Verification items for the finished model (mm, model axes). Coordinates: 2 decimals unless noted, no trailing zeros. Loops run counter-clockwise (first coordinate to the right, second up) from the corner with the lowest first, then second, coordinate; pieces in that order, holes last.
Q1. Sectioned sample at B-B (z = 13.5). Enter the section's corners in (x, y), then the cut area to 3 significant figures.
Q2. Sectioned sample at A-A (x = -22.5). Enter the section's corners in (y, z), then the cut area to 3 significant figures.
Q3. Material ranges on probe 1 along Z at (x, y) = (-3, 1.65); probe 2 along X at (y, z) = (1, -12.5); probe 3 along X at (y, z) = (1.75, 16), recorded low to high.
Q4. Go/stop test with flat-tipped pins: P1, Ø0.5, axis at y = 1.5, z = 18, coming from the +X side; P2, Ø0.6, axis at x = -33, y = 0.5, coming from the -Z side; P3, Ø1, axis at y = 0.5, z = 7.5, coming from the -X side. Record where each tip stops, or that it passes through.
Autodesk Inventor part; units mm, degrees
ref_plane "YZ Plane" through (0, 0, 0) normal (1, 0, 0) x (0, 1, 0)
ref_plane "XZ Plane" through (0, 0, 0) normal (0, 1, 0) x (-1, 0, 0)
ref_plane "XY Plane" through (0, 0, 0) normal (0, 0, 1) x (1, 0, 0)
sketch "Эскиз1" plane through (0, 0, 0) normal (0, 1, 0) x (-1, 0, 0)
  line L0 (-34.5, 19) -> (34.5, 19)
  line L1 (34.5, 19) -> (34.5, -19)
  line L2 (34.5, -19) -> (-34.5, -19)
  line L3 (-34.5, -19) -> (-34.5, 19)
  line L4 (-34.5, 19) -> (34.5, -19) construction
  line L5 (34.5, 19) -> (-34.5, -19) construction
  line L6 (34.5, -9.5) -> (34.5, 9.5)
  line L7 (36.5, -15.5) -> (32.5, -15.5)
  line L8 (32.5, -15.5) -> (32.5, -3.5)
  line L9 (32.5, -3.5) -> (36.5, -3.5)
  line L10 (36.5, -3.5) -> (36.5, -15.5)
  line L11 (36.5, -15.5) -> (32.5, -3.5) construction
  line L12 (32.5, -15.5) -> (36.5, -3.5) construction
  line L13 (36.5, 3.5) -> (32.5, 3.5)
  line L14 (32.5, 3.5) -> (32.5, 15.5)
  line L15 (32.5, 15.5) -> (36.5, 15.5)
  line L16 (36.5, 15.5) -> (36.5, 3.5)
  line L17 (36.5, 3.5) -> (32.5, 15.5) construction
  line L18 (32.5, 3.5) -> (36.5, 15.5) construction
  line L19 (-34.5, -9.5) -> (-34.5, 9.5)
  line L20 (-32.5, -15.5) -> (-36.5, -15.5)
  line L21 (-36.5, -15.5) -> (-36.5, -3.5)
  line L22 (-36.5, -3.5) -> (-32.5, -3.5)
  line L23 (-32.5, -3.5) -> (-32.5, -15.5)
  line L24 (-32.5, -15.5) -> (-36.5, -3.5) construction
  line L25 (-36.5, -15.5) -> (-32.5, -3.5) construction
  line L26 (-32.5, 3.5) -> (-36.5, 3.5)
  line L27 (-36.5, 3.5) -> (-36.5, 15.5)
  line L28 (-36.5, 15.5) -> (-32.5, 15.5)
  line L29 (-32.5, 15.5) -> (-32.5, 3.5)
  line L30 (-32.5, 3.5) -> (-36.5, 15.5) construction
  line L31 (-36.5, 3.5) -> (-32.5, 15.5) construction
  point P0 (0, 0)
  point P1 (34.5, 0)
  point P2 (-34.5, 0)
  point P3 (-34.5, 15.5)
  point P4 (-34.5, 3.5)
  point P5 (-34.5, -3.5)
  point P6 (-34.5, -15.5)
  point P7 (34.5, -15.5)
  point P8 (34.5, -3.5)
  point P9 (34.5, 3.5)
  point P10 (34.5, 15.5)
  dimension "d0" = 69
  dimension "d1" = 38
  dimension "d4" = 19
  dimension "d5" = 4
  dimension "d6" = 12
  dimension "d7" = 4
  dimension "d8" = 12
  dimension "d9" = 19
  dimension "d10" = 4
  dimension "d11" = 12
  dimension "d12" = 4
  dimension "d13" = 12
extrude "Выдавливание1" add sketch "Эскиз1" along normal blind 2 contours L0 L1 L15 L14 L13 L9 L8 L7 L2 L3 L20 L23 L22 L26 L29 L28
fillet "Сопряжение1" radius 0.5 8 edges at (-32.5, 1, -3.5) (-32.5, 1, -15.5) (-32.5, 1, 3.5) (-32.5, 1, 15.5) (32.5, 1, -15.5) (32.5, 1, -3.5) (32.5, 1, 3.5) (32.5, 1, 15.5)
fillet "Сопряжение2" radius 1 8 edges at (34.5, 1, -3.5) (34.5, 1, 3.5) (34.5, 1, -15.5) (34.5, 1, 15.5) (-34.5, 1, -15.5) (-34.5, 1, -3.5) (-34.5, 1, 3.5) (-34.5, 1, 15.5)
fillet "Сопряжение3" radius 2 4 edges at (-34.5, 1, -19) (-34.5, 1, 19) (34.5, 1, -19) (34.5, 1, 19)
sketch "Эскиз2" plane through (0, 2, 0) normal (0, 1, 0) x (1, 0, 0)
  line L0 (-34.5, -19) -> (34.5, -19)
  line L1 (34.5, -19) -> (34.5, 19)
  line L2 (34.5, 19) -> (-34.5, 19)
  line L3 (-34.5, 19) -> (-34.5, -19)
  line L4 (-34.5, -19) -> (34.5, 19) construction
  line L5 (34.5, -19) -> (-34.5, 19) construction
  line L6 (34.5, -2.5) -> (34.5, 2.5)
  line L7 (34.5, 0) -> (19.5, 0)
  line L8 (19.5, 5) -> (19.5, -5)
  line L9 (34.5, -19) -> (4.5, -19)
  line L10 (-32.5, -19) -> (32.5, -19)
  line L11 (4.5, -19) -> (4.5, -14)
  point P0 (0, 0)
  dimension "d17" = 69
  dimension "d18" = 38
  dimension "d19" = 15
  dimension "d20" = 10
  dimension "d21" = 30
  dimension "d22" = 5
sketch "Эскиз3" plane through (0, 2, 0) normal (0, 1, 0) x (1, 0, 0)
  arc A0 (32.5, -19) -> (34.5, -17) centre (32.5, -17) ccw
  line L0 (34.5, -17) -> (34.5, -16.5)
  arc A1 (34.5, -16.5) -> (33.5, -15.5) centre (33.5, -16.5) ccw
  line L1 (33.5, -15.5) -> (33, -15.5)
  arc A2 (32.5, -15) -> (33, -15.5) centre (33, -15) ccw
  line L2 (32.5, -15) -> (32.5, -4)
  arc A3 (33, -3.5) -> (32.5, -4) centre (33, -4) ccw
  line L3 (33, -3.5) -> (33.5, -3.5)
  arc A4 (33.5, -3.5) -> (34.5, -2.5) centre (33.5, -2.5) ccw
  line L4 (34.5, -2.5) -> (34.5, 2.5)
  arc A5 (34.5, 2.5) -> (33.5, 3.5) centre (33.5, 2.5) ccw
  line L5 (33.5, 3.5) -> (33, 3.5)
  arc A6 (32.5, 4) -> (33, 3.5) centre (33, 4) ccw
  line L6 (32.5, 4) -> (32.5, 15)
  arc A7 (33, 15.5) -> (32.5, 15) centre (33, 15) ccw
  line L7 (33, 15.5) -> (33.5, 15.5)
  arc A8 (33.5, 15.5) -> (34.5, 16.5) centre (33.5, 16.5) ccw
  line L8 (34.5, 16.5) -> (34.5, 17)
  arc A9 (34.5, 17) -> (32.5, 19) centre (32.5, 17) ccw
  line L9 (32.5, 19) -> (-32.5, 19)
  arc A10 (-32.5, 19) -> (-34.5, 17) centre (-32.5, 17) ccw
  line L10 (-34.5, 17) -> (-34.5, 16.5)
  arc A11 (-34.5, 16.5) -> (-33.5, 15.5) centre (-33.5, 16.5) ccw
  line L11 (-33.5, 15.5) -> (-33, 15.5)
  arc A12 (-32.5, 15) -> (-33, 15.5) centre (-33, 15) ccw
  line L12 (-32.5, 15) -> (-32.5, 4)
  arc A13 (-33, 3.5) -> (-32.5, 4) centre (-33, 4) ccw
  line L13 (-33, 3.5) -> (-33.5, 3.5)
  arc A14 (-33.5, 3.5) -> (-34.5, 2.5) centre (-33.5, 2.5) ccw
  line L14 (-34.5, 2.5) -> (-34.5, -2.5)
  arc A15 (-34.5, -2.5) -> (-33.5, -3.5) centre (-33.5, -2.5) ccw
  line L15 (-33.5, -3.5) -> (-33, -3.5)
  arc A16 (-32.5, -4) -> (-33, -3.5) centre (-33, -4) ccw
  line L16 (-32.5, -4) -> (-32.5, -15)
  arc A17 (-33, -15.5) -> (-32.5, -15) centre (-33, -15) ccw
  line L17 (-33, -15.5) -> (-33.5, -15.5)
  arc A18 (-33.5, -15.5) -> (-34.5, -16.5) centre (-33.5, -16.5) ccw
  line L18 (-34.5, -16.5) -> (-34.5, -17)
  arc A19 (-34.5, -17) -> (-32.5, -19) centre (-32.5, -17) ccw
  line L19 (-32.5, -19) -> (32.5, -19)
  circle A20 centre (-22.5, 17.35) radius 1.5
  circle A21 centre (-22.5, -17.35) radius 1.5
  circle A22 centre (-22.5, -17.35) radius 1.1
  circle A23 centre (-22.5, 17.35) radius 1.1
  line L20 (32.5, 19) -> (-32.5, 19)
  line L21 (-32.5, -19) -> (32.5, -19)
  line L22 (-23.6, 19) -> (-21.4, 19)
  line L23 (-21.4, 19) -> (-21.4, -19)
  line L24 (-21.4, -19) -> (-23.6, -19)
  line L25 (-23.6, -19) -> (-23.6, 19)
  point P0 (0, 0)
  point P1 (-23.6, 16.3302)
  point P2 (-21.4, 16.3302)
  point P3 (-21.4, -19)
  point P4 (-21.4, -16.3302)
  point P5 (-23.6, -16.3302)
  point P6 (-23.6, -17.35)
  point P7 (-21.4, -17.35)
  point P8 (-23.6, 17.35)
  point P9 (-21.4, 17.35)
  dimension "d23" = 2.2
  dimension "d24" = 2.2
extrude "Выдавливание2" cut sketch "Эскиз3" against normal blind 10 contours L19 L25 A21 L23 | A21 L25 A22 L23 | A22 | L25 L9 L23 A20 | A20 L23 A23 L25 | A23 picked at (-22.5442, -18.7071) picked at (-22.5442, 18.7071)
fillet "Сопряжение4" radius 1 4 edges at (-23.6, 1, 19) (-21.4, 1, 19) (-23.6, 1, -19) (-21.4, 1, -19)
mirror "Зеркальное отражение1" about plane through (0, 0, 0) normal (1, 0, 0) of "Выдавливание2", "Сопряжение4"
sketch "Эскиз4" plane through (0, 2, 0) normal (0, 1, 0) x (1, 0, 0)
  arc A0 (-14, 18.7) -> (-14.3, 19) centre (-14.3, 18.7) ccw
  line L0 (-14.3, 19) -> (-26, 19)
  arc A1 (-26, 19) -> (-28, 17) centre (-26, 17) ccw
  line L1 (-28, 17) -> (-28, -17)
  arc A2 (-28, -17) -> (-26, -19) centre (-26, -17) ccw
  line L2 (-26, -19) -> (8, -19)
  arc A3 (8, -19) -> (10, -17) centre (8, -17) ccw
  line L3 (10, -17) -> (10, 17)
  arc A4 (10, 17) -> (8, 19) centre (8, 17) ccw
  line L4 (8, 19) -> (-1.7, 19)
  arc A5 (-1.7, 19) -> (-2, 18.7) centre (-1.7, 18.7) ccw
  line L5 (-2, 18.7) -> (-2, 18.3)
  arc A6 (-2.3, 18) -> (-2, 18.3) centre (-2.3, 18.3) ccw
  line L6 (-2.3, 18) -> (-13.7, 18)
  arc A7 (-14, 18.3) -> (-13.7, 18) centre (-13.7, 18.3) ccw
  line L7 (-14, 18.3) -> (-14, 18.7)
  arc A8 (21.4, 18) -> (20.4, 19) centre (20.4, 18) ccw
  line L8 (20.4, 19) -> (-20.4, 19)
  arc A9 (-20.4, 19) -> (-21.4, 18) centre (-20.4, 18) ccw
  line L9 (-21.4, 18) -> (-21.4, 17.35)
  arc A10 (-23.6, 17.35) -> (-21.4, 17.35) centre (-22.5, 17.35) ccw
  line L10 (-23.6, 17.35) -> (-23.6, 18)
  arc A11 (-23.6, 18) -> (-24.6, 19) centre (-24.6, 18) ccw
  line L11 (-24.6, 19) -> (-32.5, 19)
  arc A12 (-32.5, 19) -> (-34.5, 17) centre (-32.5, 17) ccw
  line L12 (-34.5, 17) -> (-34.5, 16.5)
  arc A13 (-34.5, 16.5) -> (-33.5, 15.5) centre (-33.5, 16.5) ccw
  line L13 (-33.5, 15.5) -> (-33, 15.5)
  arc A14 (-32.5, 15) -> (-33, 15.5) centre (-33, 15) ccw
  line L14 (-32.5, 15) -> (-32.5, 4)
  arc A15 (-33, 3.5) -> (-32.5, 4) centre (-33, 4) ccw
  line L15 (-33, 3.5) -> (-33.5, 3.5)
  arc A16 (-33.5, 3.5) -> (-34.5, 2.5) centre (-33.5, 2.5) ccw
  line L16 (-34.5, 2.5) -> (-34.5, -2.5)
  arc A17 (-34.5, -2.5) -> (-33.5, -3.5) centre (-33.5, -2.5) ccw
  line L17 (-33.5, -3.5) -> (-33, -3.5)
  arc A18 (-32.5, -4) -> (-33, -3.5) centre (-33, -4) ccw
  line L18 (-32.5, -4) -> (-32.5, -15)
  arc A19 (-33, -15.5) -> (-32.5, -15) centre (-33, -15) ccw
  line L19 (-33, -15.5) -> (-33.5, -15.5)
  arc A20 (-33.5, -15.5) -> (-34.5, -16.5) centre (-33.5, -16.5) ccw
  line L20 (-34.5, -16.5) -> (-34.5, -17)
  arc A21 (-34.5, -17) -> (-32.5, -19) centre (-32.5, -17) ccw
  line L21 (-32.5, -19) -> (-24.6, -19)
  arc A22 (-24.6, -19) -> (-23.6, -18) centre (-24.6, -18) ccw
  line L22 (-23.6, -18) -> (-23.6, -17.35)
  arc A23 (-21.4, -17.35) -> (-23.6, -17.35) centre (-22.5, -17.35) ccw
  line L23 (-21.4, -17.35) -> (-21.4, -18)
  arc A24 (-21.4, -18) -> (-20.4, -19) centre (-20.4, -18) ccw
  line L24 (-20.4, -19) -> (20.4, -19)
  arc A25 (20.4, -19) -> (21.4, -18) centre (20.4, -18) ccw
  line L25 (21.4, -18) -> (21.4, -17.35)
  arc A26 (23.6, -17.35) -> (21.4, -17.35) centre (22.5, -17.35) ccw
  line L26 (23.6, -17.35) -> (23.6, -18)
  arc A27 (23.6, -18) -> (24.6, -19) centre (24.6, -18) ccw
  line L27 (24.6, -19) -> (32.5, -19)
  arc A28 (32.5, -19) -> (34.5, -17) centre (32.5, -17) ccw
  line L28 (34.5, -17) -> (34.5, -16.5)
  arc A29 (34.5, -16.5) -> (33.5, -15.5) centre (33.5, -16.5) ccw
  line L29 (33.5, -15.5) -> (33, -15.5)
  arc A30 (32.5, -15) -> (33, -15.5) centre (33, -15) ccw
  line L30 (32.5, -15) -> (32.5, -4)
  arc A31 (33, -3.5) -> (32.5, -4) centre (33, -4) ccw
  line L31 (33, -3.5) -> (33.5, -3.5)
  arc A32 (33.5, -3.5) -> (34.5, -2.5) centre (33.5, -2.5) ccw
  line L32 (34.5, -2.5) -> (34.5, 2.5)
  arc A33 (34.5, 2.5) -> (33.5, 3.5) centre (33.5, 2.5) ccw
  line L33 (33.5, 3.5) -> (33, 3.5)
  arc A34 (32.5, 4) -> (33, 3.5) centre (33, 4) ccw
  line L34 (32.5, 4) -> (32.5, 15)
  arc A35 (33, 15.5) -> (32.5, 15) centre (33, 15) ccw
  line L35 (33, 15.5) -> (33.5, 15.5)
  arc A36 (33.5, 15.5) -> (34.5, 16.5) centre (33.5, 16.5) ccw
  line L36 (34.5, 16.5) -> (34.5, 17)
  arc A37 (34.5, 17) -> (32.5, 19) centre (32.5, 17) ccw
  line L37 (32.5, 19) -> (24.6, 19)
  arc A38 (24.6, 19) -> (23.6, 18) centre (24.6, 18) ccw
  line L38 (23.6, 18) -> (23.6, 17.35)
  arc A39 (21.4, 17.35) -> (23.6, 17.35) centre (22.5, 17.35) ccw
  line L39 (21.4, 17.35) -> (21.4, 18)
  point P0 (0, 0)
extrude "Выдавливание3" cut sketch "Эскиз4" against normal blind 10 contours A0 L8 A5 L5 A6 L6 A7 L7
properties part number "BMS_board"
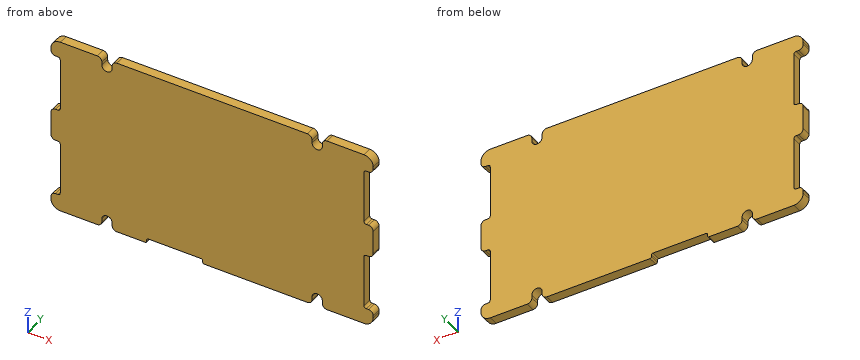
Geometry check:
1. outline: (-32.5, 0) - (32.5, 0) - (32.5, 2) - (-32.5, 2) - close
1. area: 130 mm2
2. outline: (0, -16.25) - (2, -16.25) - (2, 16.25) - (0, 16.25) - close
2. area: 65.0 mm2
3. probe 1: z = -18 to 19
3. probe 2: x = -32.5 to 32.5
3. probe 3: x = -34.37 to 34.37
4. P1: stops at x = 34.35
4. P2: stops at z = -18.99
4. P3: stops at x = -32.5
